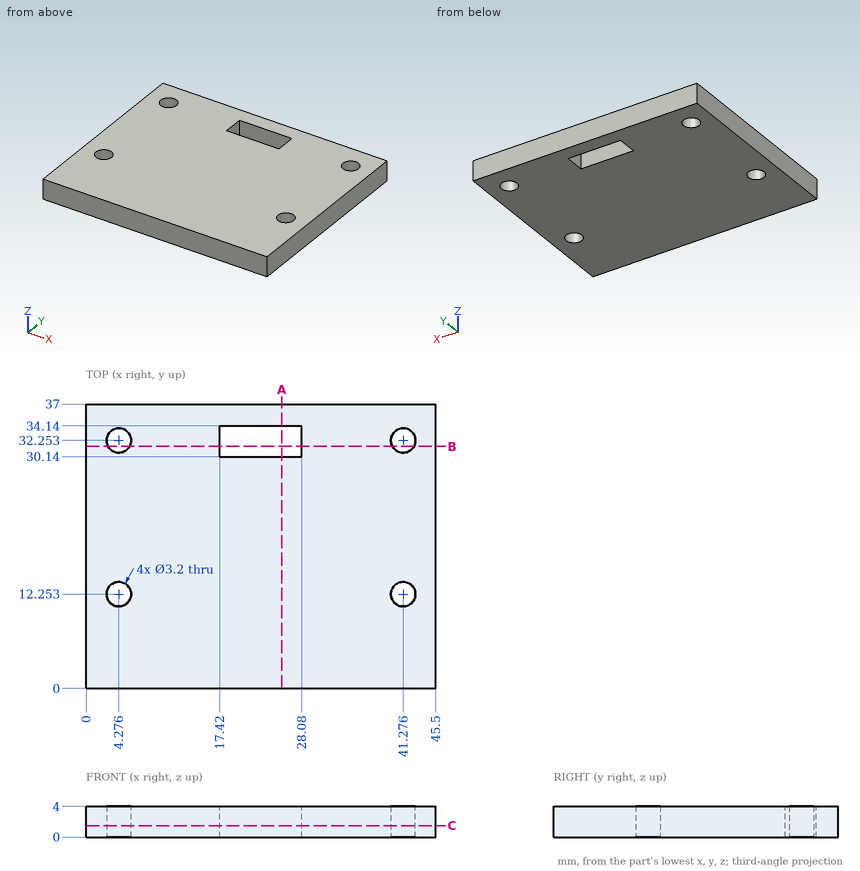
Geometry: see drawing. Coordinates: mm, zero at the bounding-box minimum. Round coordinates to 2 decimals unless told otherwise and drop trailing zeros. Loops run counter-clockwise (first coordinate to the right, second up) from the corner with the lowest first, then second, coordinate; pieces in that order, holes last. Notation, with made-up numbers: (-2.5, -31.75) -> (50.5, -31.75) arc R21 ccw to (50.5, -3.75) -> close; hole circle Ø9 at (-17.5, 57). An arc over 180 degrees is marked (long way). One line per question, with ' | ' between items. Start each with the question number.
1. Section A-A on x = 25.5. Output: boundary loops of the cut face in (y, z).
2. Line query: line 1 along Y through (x, z) = (18, 0.9); line 2 along X through (y, z) = (13, 2.15); line 3 along X through (y, z) = (34, 3). Output: solid intervals per line, ascending. Write a range as [from, to].
3. Section C-C on z = 1.5. Output: boundary loops of the cut face in (x, y).
4. Section B-B on y = 31.5. Output: boundary loops of the cut face in (x, z), and give its area (3 significant figures).
5. Contact query for a flat-ended pin moving along its axis: pin 1 (2.5 mm diameter, centred on x = 41.28, y = 32.25, fed in from +Z). Output: stop coordinate, or through.
Returned:
1) outline: (0, 0) -> (30.14, 0) -> (30.14, 4) -> (0, 4) -> close; (34.14, 0) -> (37, 0) -> (37, 4) -> (34.14, 4) -> close
2) line 1: y = [0, 30.14], [34.14, 37] | line 2: x = [0, 2.86], [5.69, 39.86], [42.69, 45.5] | line 3: x = [0, 17.42], [28.08, 45.5]
3) outline: (0, 0) -> (45.5, 0) -> (45.5, 37) -> (0, 37) -> close; hole circle Ø3.2 at (4.28, 12.25); hole circle Ø3.2 at (4.28, 32.25); hole (17.42, 30.14) -> (28.08, 30.14) -> (28.08, 34.14) -> (17.42, 34.14) -> close; hole circle Ø3.2 at (41.28, 12.25); hole circle Ø3.2 at (41.28, 32.25)
4) outline: (0, 0) -> (2.86, 0) -> (2.86, 4) -> (0, 4) -> close; (5.69, 0) -> (17.42, 0) -> (17.42, 4) -> (5.69, 4) -> close; (28.08, 0) -> (39.86, 0) -> (39.86, 4) -> (28.08, 4) -> close; (42.69, 0) -> (45.5, 0) -> (45.5, 4) -> (42.69, 4) -> close | area: 117 mm2
5) pin 1: passes through
